```python
from build123d import *

# Parameters (mm, degrees)
F1_DEPTH = 8.89


with BuildPart() as f1:
    # F0 (on Top) → F1 (new body)
    with BuildSketch(Plane.XY):
        Polygon((38.373657, 41.128395), (-10.907251, 41.128395), (-38.281802, 41.128395), (-38.281802, 4.189338), (-38.281802, -37.003323), (38.373657, -37.003323), (38.373657, -3.794326), (76.488459, -3.794326), (76.488459, 3.317674), (76.488459, 10.429674), (38.373657, 10.429674), align=None)
        with BuildLine():
            Line((-16.520221, 7.932111), (-10.907251, 13.545081))
            Line((-10.907251, 13.545081), (-7.36036, 17.091973))
            Line((-7.36036, 17.091973), (-7.36036, 30.459993))
            ThreePointArc((-7.36036, 30.459993), (0.25965, 38.079973), (7.87964, 30.459973))
            Line((7.87964, 30.459973), (7.87964, 17.091973))
            ThreePointArc((7.87964, 17.091973), (6.719564, 11.259877), (3.415948, 6.315665))
            Line((3.415948, 6.315665), (-5.739092, -2.839375))
            Line((-5.739092, -2.839375), (-14.898953, -11.999236))
            Line((-14.898953, -11.999236), (-14.898953, -25.367236))
            ThreePointArc((-14.898953, -25.367236), (-22.518953, -32.987236), (-30.138953, -25.367236))
            Line((-30.138953, -25.367236), (-30.138953, -11.999235))
            ThreePointArc((-30.138953, -11.999235), (-28.978877, -6.16714), (-25.67526, -1.222928))
            Line((-25.67526, -1.222928), (-16.520221, 7.932111))
        make_face(mode=Mode.SUBTRACT)
    extrude(amount=F1_DEPTH)


solid = f1.part
```
Design review of the part built by this model. Coordinates are the model's own, in mm. A direction names the side the tool comes from. Give positions to 0.01 mm unless a question says otherwise; leave off trailing zeros. Write each loop counter-clockwise with the first axis right and the second up, starting at its lowest first coordinate (ties: lowest second). Pieces come first, ordered by that corner, then holes.
(1) Tool access review of faces 5 (the face through (-29.01, -6.24, 4.38)), 6 (the face through (38.374, -21, 4)), 7 (the face through (58, 10.43, 4)): name each direction out of +Z, -Z, +X, -X, +Y, -Y from which nothing blocks a thin tool from reaching the whole face with its end or side.
Checked values:
face 5: +Z, -Z
face 6: +Z, -Z, +X, -Y
face 7: +Z, -Z, +X, +Y
(2) Wall thickness on line 1 along X through (y, z) = (-19, 3.25); line 2 along X through (y, z) = (26.5, 6.25); line 3 along Y through (x, z) = (6, 4.25): over which ranges is each line inside the solid? List them lowest first.
Checked values:
line 1: x = -38.28 to -30.14, -14.9 to 38.37
line 2: x = -38.28 to -7.36, 7.88 to 38.37
line 3: y = -37 to 9.76, 35.47 to 41.13
(3) Add section C-C (z = 5.75). Give the boundary of the cut face in (x, y).
Checked values:
outline: (-38.28, -37) - (38.37, -37) - (38.37, -3.79) - (76.49, -3.79) - (76.49, 10.43) - (38.37, 10.43) - (38.37, 41.13) - (-38.28, 41.13) - close; hole (-30.14, -25.37) arc R7.62 ccw to (-14.9, -25.37) - (-14.9, -12) - (3.42, 6.32) arc R15.24 ccw to (7.88, 17.09) - (7.88, 30.46) arc R7.62 ccw to (-7.36, 30.46) - (-7.36, 17.09) - (-10.91, 13.55) - (-25.68, -1.22) arc R15.24 ccw to (-30.14, -12) - close
(4) Clearance check with flat-ended pins moving along their axes: pin 1 Ø4.5 at (y, z) = (-27.5, 2.5) entering from +X; pin 2 Ø5 at (x, z) = (60, 1) entering from -Y; pin 3 Ø2.5 at (x, z) = (59.5, 2.5) entering from +Y. State where each tip first meets the part, or that it passes through.
Checked values:
pin 1: stops at x = 38.37
pin 2: stops at y = -3.79
pin 3: stops at y = 10.43
(5) Mouldability with a two-part tool opening along Y and no side actions: class faces 1 (the face through (7.88, 24, 4)), 2 (the face through (0, -37.003, 4)), 3 (the face through (-22.351, -32.985, 4.383)), 4 (the face through (1, 41.128, 4)) as +Y half, -Y half, draft (parallel to the pull), parting line (faces both ways), or undercut.
Checked values:
face 1: undercut
face 2: -Y half
face 3: undercut
face 4: +Y half
(6) Add section D-D (x = 62.5). Give the boundary of the cut face in (y, z), and give its area (3 significant figures).
Checked values:
outline: (-3.79, 0) - (10.43, 0) - (10.43, 8.89) - (-3.79, 8.89) - close
area: 126 mm2
(7) Add section A-A (y = -19). Give the boundary of the cut face in (x, z), and give its area (3 significant figures).
Checked values:
outline: (-38.28, 0) - (-30.14, 0) - (-30.14, 8.89) - (-38.28, 8.89) - close; (-14.9, 0) - (38.37, 0) - (38.37, 8.89) - (-14.9, 8.89) - close
area: 546 mm2
(8) Add section B-B (x = -23). Give the boundary of the cut face in (y, z).
Checked values:
outline: (-37, 0) - (-32.97, 0) - (-32.97, 8.89) - (-37, 8.89) - close; (1.45, 0) - (41.13, 0) - (41.13, 8.89) - (1.45, 8.89) - close
